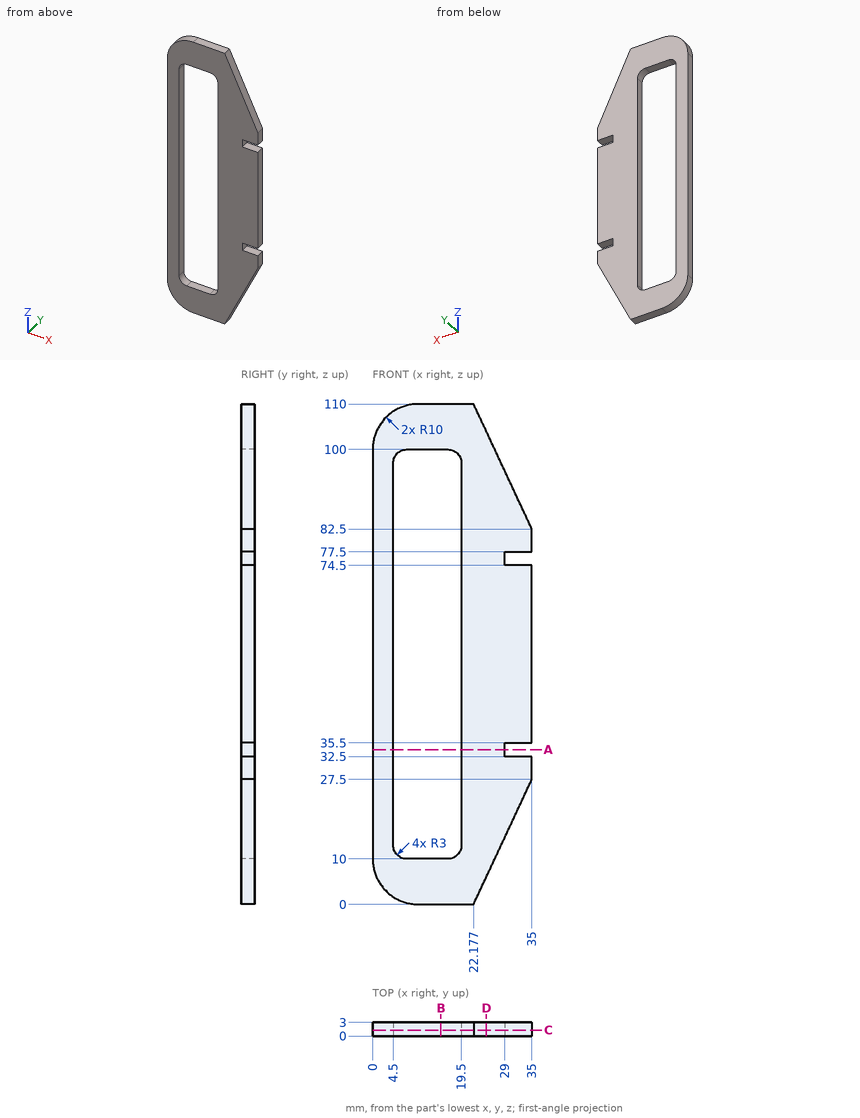
Print and shaded views of the part. All mm, measured from the part's lowest x, y and z. Coordinates: 2 decimals unless noted, no trailing zeros. Write each loop counter-clockwise with the first axis right and the second up, starting at its lowest first coordinate (ties: lowest second). Pieces come first, ordered by that corner, then holes. Notation, with made-up numbers: (-33, -5.75) -> (3, -5.75) arc R20 cw to (3, 0.25) -> close; hole circle Ø4 at (70.5, -29). An arc over 180 degrees is marked (long way). Use CSV: the item, a comma, the result in double quotes. Start each with the question number.
Q1. Cut at D-D, the plane x = 25. List the corners of the cut face in (y, z) (1 decimal).
Q2. Flat gauge pins, fed straight in: pin 1 Ø1.5 at (y, z) = (1.5, 33.5) entering from +X; pin 2 Ø0.9 at (x, y) = (30.5, 1) entering from +Z (1 decimal); pin 3 Ø1.5 at (x, y) = (31.5, 1.5) entering from -Z (1 decimal). Where does each tip first touch, or does it go through?
Q3. Drill centre lines: probe 1 along X at (y, z) = (1.5, 42); probe 2 along Z at (x, y) = (14, 2.75); probe 3 along Z at (x, y) = (31, 2.25) (1 decimal). Where is each one in solid material? Low to high.
Q4. Cut at A-A, the plane z = 34. List the corners of the cut face in (x, y), then the cut area to 3 significant figures.
Q5. Cut at B-B, the plane x = 15. List the corners of the cut face in (y, z).
Q6. Cut at C-C, the plane y = 1.3. List the corners of the cut face in (x, z), then the cut area to 3 significant figures.
Checked values:
1,outline,"(0, 6.1) -> (3, 6.1) -> (3, 103.9) -> (0, 103.9) -> close"
2,pin 1,"stops at x = 29"
2,pin 2,"stops at z = 93.1"
2,pin 3,"stops at z = 18.4"
3,probe 1,"x = 0 to 4.5, 19.5 to 35"
3,probe 2,"z = 0 to 10, 100 to 110"
3,probe 3,"z = 18.9 to 32.5, 35.5 to 74.5, 77.5 to 91.1"
4,outline,"(0, 0) -> (4.5, 0) -> (4.5, 3) -> (0, 3) -> close; (19.5, 0) -> (29, 0) -> (29, 3) -> (19.5, 3) -> close"
4,area,"42.0 mm²"
5,outline,"(0, 0) -> (3, 0) -> (3, 10) -> (0, 10) -> close; (0, 100) -> (3, 100) -> (3, 110) -> (0, 110) -> close"
6,outline,"(0, 10) arc R10 ccw to (10, 0) -> (22.18, 0) -> (35, 27.5) -> (35, 32.5) -> (29, 32.5) -> (29, 35.5) -> (35, 35.5) -> (35, 74.5) -> (29, 74.5) -> (29, 77.5) -> (35, 77.5) -> (35, 82.5) -> (22.18, 110) -> (10, 110) arc R10 ccw to (0, 100) -> close; hole (4.5, 13) arc R3 ccw to (7.5, 10) -> (16.5, 10) arc R3 ccw to (19.5, 13) -> (19.5, 97) arc R3 ccw to (16.5, 100) -> (7.5, 100) arc R3 ccw to (4.5, 97) -> close"
6,area,"2,080 mm²"
